Design review of the part shown in the three views and the two pictorial views. Dimensions are in mm from the part's minimum x, y and z. A direction names the side the tool comes from. Round coordinates to 2 decimals unless told otherwise and drop trailing zeros. Loops run counter-clockwise (first coordinate to the right, second up) from the corner with the lowest first, then second, coordinate; pieces in that order, holes last.
1) Take a section at C-C (x = 1.5). State the section outline as (y, z) points, then the cut area to 3 significant figures.
2) Take a section at B-B (z = 7.5). State the section outline as (x, y) points, then the cut area to 3 significant figures.
3) Take a section at A-A (y = 9). State the section outline as (x, z) points.
4) Tool access review of the marked faces 1, 2 and 3: name each direction out of +Z, -Z, +X, -X, +Y, -Y from which nothing blocks a thin tool from reaching the whole face with its end or side.
5) Insertion check: pin 1 (6.5 mm diameter, centred on x = 2.5, y = 8, fed in from +Z). The pin has a flat end and moves straight along its axis. Give the tip position at first contact, or say it passes through.
6) Wall thickness on L1, parallel to Z at x = 19.25, y = 11; L2, parallel to X at y = 4.75, z = 8.25: over which ranges is each line inside the solid? List them lowest first.
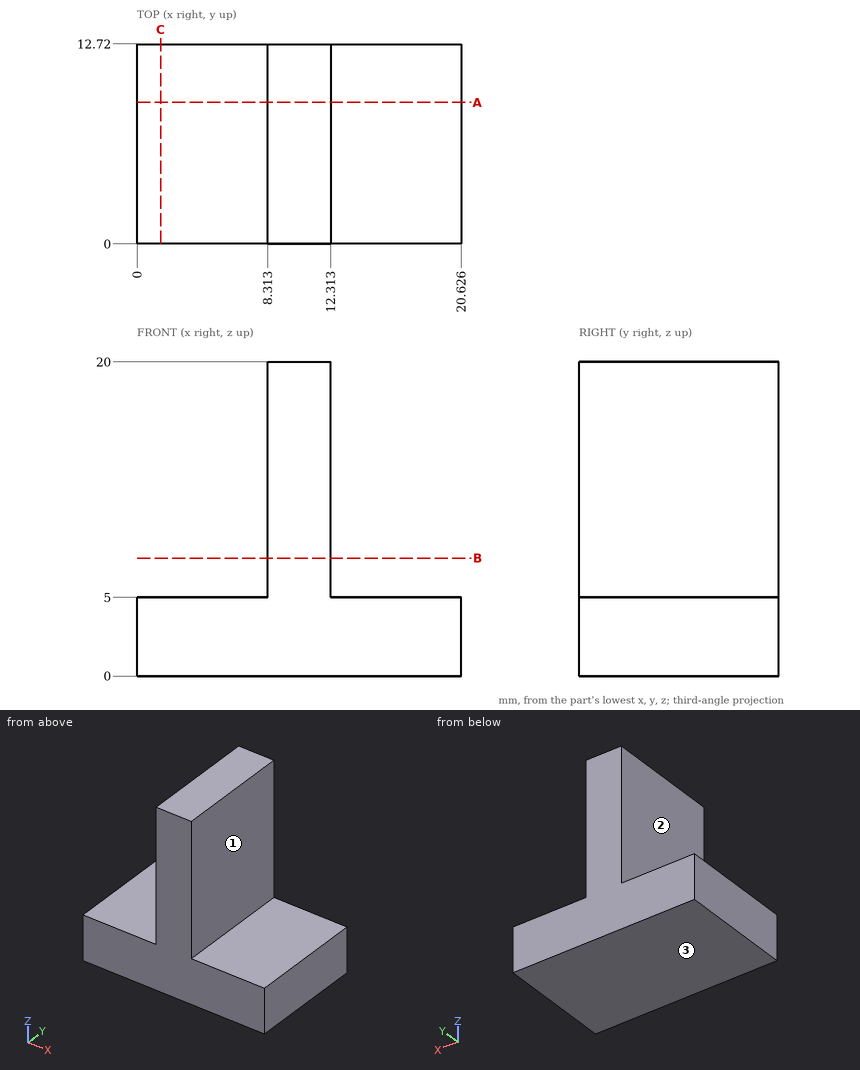
Response:
1. outline: (0, 0) - (12.72, 0) - (12.72, 5) - (0, 5) - close
1. area: 63.6 mm2
2. outline: (8.31, 0) - (12.31, 0) - (12.31, 12.72) - (8.31, 12.72) - close
2. area: 50.9 mm2
3. outline: (0, 0) - (20.63, 0) - (20.63, 5) - (12.31, 5) - (12.31, 20) - (8.31, 20) - (8.31, 5) - (0, 5) - close
4. face 1: +Z, +X, +Y, -Y
4. face 2: +Z, -X, +Y, -Y
4. face 3: -Z, +X, -X, +Y, -Y
5. pin 1: stops at z = 5
6. L1: z = 0 to 5
6. L2: x = 8.31 to 12.31
